Work out the finished part from the listing and answer in its coordinate system (mm). Give positions to 0.01 mm unless a question says otherwise; leave off trailing zeros. Loops run counter-clockwise (first coordinate to the right, second up) from the corner with the lowest first, then second, coordinate; pieces in that order, holes last. Notation, with made-up numbers: (71, 34) - (126, 34) arc R17 cw to (126, 56) - close; hole circle Ø4 at (-2.5, 81). An arc over 180 degrees is marked (long way). One line per question, with ' | ' between items.
from build123d import *

# Parameters (mm, degrees)
F0_W     = 479.425
F0_H     = 66.675
F1_DEPTH = 3.175
F2_W     = 3.175
F2_H     = 9.525
F3_DEPTH = 3.176
F4_W     = 9.525
F4_H     = 3.175
F5_DEPTH = 3.176


with BuildPart() as f1:
    # F0 (on Front) → F1 (new body)
    with BuildSketch(Plane.XZ):
        Rectangle(F0_W, F0_H)
    extrude(amount=F1_DEPTH)

    # F2 (on face) → F3 (cut, through all)
    with BuildSketch(Plane.XZ.offset(3.175)):
        with Locations((-238.125, -28.575)):
            Rectangle(F2_W, F2_H)
        with Locations((-238.125, -9.525)):
            Rectangle(F2_W, F2_H)
        with Locations((-238.125, 9.525)):
            Rectangle(F2_W, F2_H)
        with Locations((-238.125, 28.575)):
            Rectangle(F2_W, F2_H)
        with Locations((-158.75, -28.575)):
            Rectangle(F2_W, F2_H)
        with Locations((-158.75, -9.525)):
            Rectangle(F2_W, F2_H)
        with Locations((-158.75, 9.525)):
            Rectangle(F2_W, F2_H)
        with Locations((-158.75, 28.575)):
            Rectangle(F2_W, F2_H)
        with Locations((-79.375, -28.575)):
            Rectangle(F2_W, F2_H)
        with Locations((-79.375, -9.525)):
            Rectangle(F2_W, F2_H)
        with Locations((-79.375, 9.525)):
            Rectangle(F2_W, F2_H)
        with Locations((-79.375, 28.575)):
            Rectangle(F2_W, F2_H)
        with Locations((0, -28.575)):
            Rectangle(F2_W, F2_H)
        with Locations((0, -9.525)):
            Rectangle(F2_W, F2_H)
        with Locations((0, 9.525)):
            Rectangle(F2_W, F2_H)
        with Locations((0, 28.575)):
            Rectangle(F2_W, F2_H)
        with Locations((79.375, -28.575)):
            Rectangle(F2_W, F2_H)
        with Locations((79.375, -9.525)):
            Rectangle(F2_W, F2_H)
        with Locations((79.375, 9.525)):
            Rectangle(F2_W, F2_H)
        with Locations((79.375, 28.575)):
            Rectangle(F2_W, F2_H)
        with Locations((158.75, -28.575)):
            Rectangle(F2_W, F2_H)
        with Locations((158.75, -9.525)):
            Rectangle(F2_W, F2_H)
        with Locations((158.75, 9.525)):
            Rectangle(F2_W, F2_H)
        with Locations((158.75, 28.575)):
            Rectangle(F2_W, F2_H)
        with Locations((238.125, -28.575)):
            Rectangle(F2_W, F2_H)
        with Locations((238.125, -9.525)):
            Rectangle(F2_W, F2_H)
        with Locations((238.125, 9.525)):
            Rectangle(F2_W, F2_H)
        with Locations((238.125, 28.575)):
            Rectangle(F2_W, F2_H)
    extrude(amount=-F3_DEPTH, mode=Mode.SUBTRACT)

    # F4 (on face) → F5 (cut, through all)
    with BuildSketch(Plane.XZ.offset(3.175)):
        with Locations((-219.075, -31.75)):
            Rectangle(F4_W, F4_H)
        with Locations((-198.4375, -31.75)):
            Rectangle(F4_W, F4_H)
        with Locations((-177.8, -31.75)):
            Rectangle(F4_W, F4_H)
        with Locations((-139.7, -31.75)):
            Rectangle(F4_W, F4_H)
        with Locations((-119.0625, -31.75)):
            Rectangle(F4_W, F4_H)
        with Locations((-98.425, -31.75)):
            Rectangle(F4_W, F4_H)
        with Locations((-60.325, -31.75)):
            Rectangle(F4_W, F4_H)
        with Locations((-39.6875, -31.75)):
            Rectangle(F4_W, F4_H)
        with Locations((-19.05, -31.75)):
            Rectangle(F4_W, F4_H)
        with Locations((19.05, -31.75)):
            Rectangle(F4_W, F4_H)
        with Locations((39.6875, -31.75)):
            Rectangle(F4_W, F4_H)
        with Locations((60.325, -31.75)):
            Rectangle(F4_W, F4_H)
        with Locations((98.425, -31.75)):
            Rectangle(F4_W, F4_H)
        with Locations((119.0625, -31.75)):
            Rectangle(F4_W, F4_H)
        with Locations((139.7, -31.75)):
            Rectangle(F4_W, F4_H)
        with Locations((177.8, -31.75)):
            Rectangle(F4_W, F4_H)
        with Locations((198.4375, -31.75)):
            Rectangle(F4_W, F4_H)
        with Locations((219.075, -31.75)):
            Rectangle(F4_W, F4_H)
    extrude(amount=-F5_DEPTH, mode=Mode.SUBTRACT)


solid = f1.part
1. Find section A-A on y = -1.6. State how many separate pieces and enclosed holes the cut face has, then the cut area to 3 significant figures.
Evaluation:
separate pieces: 1 | enclosed holes: 10 | area: 30,600 mm2
2. Consider L1, parallel to X at y = -1.2, z = 25; L2, parallel to Z at x = -119, y = -2.4. Determine where each line is inside the solid, lowest interval first.
Evaluation:
L1: -236.54 to -160.34, -157.16 to -80.96, -77.79 to -1.59, 1.59 to 77.79, 80.96 to 157.16, 160.34 to 236.54 | L2: -30.16 to 33.34
3. Flat-ended cylindrical pins translate along their axes: pin 1 (1 mm diameter, centred on x = -79.5, y = -1, fed in from +Z); pin 2 (1 mm diameter, centred on y = -1.5, z = -31.5, fed in from -X); pin 3 (1 mm diameter, centred on x = 21, y = -1.5, fed in from -Z); pin 4 (1 mm diameter, centred on x = 99, z = 21.5, fed in from +Y). Find the tip coordinate at first contact, or state that the pin passes through.
Evaluation:
pin 1: z = 23.81 | pin 2: x = -236.54 | pin 3: z = -30.16 | pin 4: y = 0
4. Find section B-B on x = 19.5. Write down the section's boundary in (y, z) (1 decimal).
Evaluation:
outline: (-3.2, -30.2) - (0, -30.2) - (0, 33.3) - (-3.2, 33.3) - close
